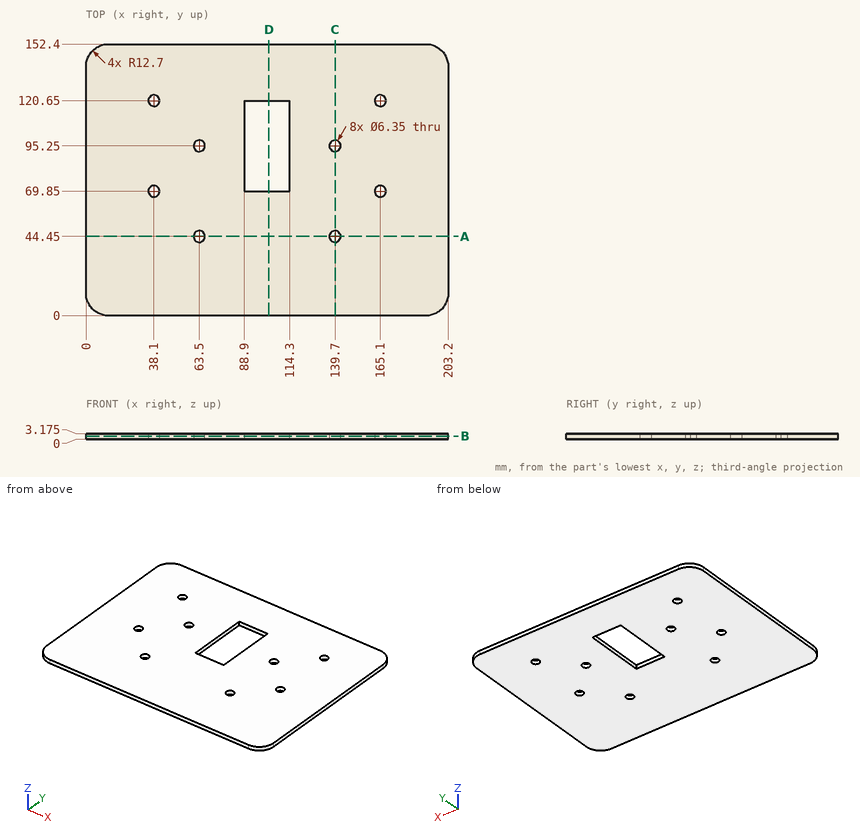
Design review of the part shown in the three views and the two pictorial views. Dimensions are in mm from the part's minimum x, y and z. Give positions to 0.01 mm unless a question says otherwise; leave off trailing zeros. Order: outer loops, then holes, each group sorted by start corner. A loop starts at its lowest first (then second) coordinate and runs counter-clockwise, first axis right, second up. Notation, with made-up numbers: (-31.75, 55.5) -> (1.25, 55.5) arc R17 ccw to (1.25, 69.5) -> close; hole circle Ø7 at (-6.5, 36.25). An arc over 180 degrees is marked (long way). Write each question's results on one line, items separated by ' | '. Start each with the question number.
Q1. Add section A-A on y = 44.45. Give the boundary of the cut face in (x, z) (3 decimals), and give its area (3 significant figures).
Q2. Wall thickness on L1, parallel to X at y = 107, z = 0.3; L2, parallel to Y at x = 38.1, z = 0.9 (3 decimals); L3, parallel to X at y = 70.5, z = 0.65: over which ranges is each line inside the solid? List them lowest first. Write a range as from..to.
Q3. Add section D-D on x = 102.5. Give the boundary of the cut face in (y, z) (3 decimals).
Q4. Add section B-B on z = 1.8. State how many separate pieces and enclosed holes the cut face has, and give its area (3 significant figures).
Q5. Add section C-C on x = 139.7. Give the boundary of the cut face in (y, z) (3 decimals), and give its area (3 significant figures).
Q6. For pin 1 (5 mm diameter, centred on x = 63.5, y = 95.25, fed in from +Z), flat-tipped, find the tip position at first contact; note if it passes through.
Found:
1) outline: (0, 0) -> (60.325, 0) -> (60.325, 3.175) -> (0, 3.175) -> close; (66.675, 0) -> (136.525, 0) -> (136.525, 3.175) -> (66.675, 3.175) -> close; (142.875, 0) -> (203.2, 0) -> (203.2, 3.175) -> (142.875, 3.175) -> close | area: 605 mm2
2) L1: x = 0..88.9, 114.3..203.2 | L2: y = 0..66.675, 73.025..117.475, 123.825..152.4 | L3: x = 0..34.99, 41.21..88.9, 114.3..161.99, 168.21..203.2
3) outline: (0, 0) -> (69.85, 0) -> (69.85, 3.175) -> (0, 3.175) -> close; (120.65, 0) -> (152.4, 0) -> (152.4, 3.175) -> (120.65, 3.175) -> close
4) separate pieces: 1 | enclosed holes: 9 | area: 29,300 mm2
5) outline: (0, 0) -> (41.275, 0) -> (41.275, 3.175) -> (0, 3.175) -> close; (47.625, 0) -> (92.075, 0) -> (92.075, 3.175) -> (47.625, 3.175) -> close; (98.425, 0) -> (152.4, 0) -> (152.4, 3.175) -> (98.425, 3.175) -> close | area: 444 mm2
6) pin 1: passes through
